Solid Edge part; units mm, degrees
sketch "Sketch1" plane through (0, 0, 0) normal (0, -1, 0) x (1, 0, 0)
  circle A0 centre (0, 0) radius 1.5
extrude "Protrusion1" add sketch "Sketch1" against normal blind 16
sketch "Sketch2" plane through (0, 16, 0) normal (0, 1, 0) x (1, 0, 0)
  circle A0 centre (0, 0) radius 3
extrude "ExtrudedProtrusion_2" add sketch "Sketch2" along normal blind 2.52
sketch "Sketch3" plane through (0, 18.52, 0) normal (0, 1, 0) x (-1, 0, 0)
  line L0 (-2.9311, 0.6393) -> (2.9311, 0.6393)
  arc A0 (2.9311, 0.6393) -> (2.9311, -0.6393) centre (0, 0) cw
  line L1 (2.9311, -0.6393) -> (-2.9311, -0.6393)
  arc A1 (-2.9311, -0.6393) -> (-2.9311, 0.6393) centre (0, 0) cw
extrude "ExtrudedCutout_1" cut sketch "Sketch3" against normal blind 0.8
cosmetic_thread "Thread1"
properties material "Nylon, general purpose"
Geometry check sheet. Reference: the model listing, model coordinates, mm. A direction names the side the tool comes from. Give positions to 0.01 mm unless a question says otherwise; leave off trailing zeros. Loops run counter-clockwise (first coordinate to the right, second up) from the corner with the lowest first, then second, coordinate; pieces in that order, holes last.
(1) Section check A-A on z = 0. Record the cut outline in (x, y), then the cut area to 3 significant figures.
From the geometry:
outline: (-3, 16) - (-1.5, 16) - (-1.5, 0) - (1.5, 0) - (1.5, 16) - (3, 16) - (3, 17.72) - (-3, 17.72) - close
area: 58.3 mm2
(2) Section check B-B on x = 2.4. Record the cut outline in (y, z).
From the geometry:
outline: (16, -1.8) - (18.52, -1.8) - (18.52, -0.64) - (17.72, -0.64) - (17.72, 0.64) - (18.52, 0.64) - (18.52, 1.8) - (16, 1.8) - close
(3) Thickness scan on L1, parallel to Y at x = 2.7, z = 0.2; L2, parallel to Y at x = -0.2, z = 1.75; L3, parallel to Z at x = 0.1, y = 8.5. Record the ranges inside material, lowest first.
From the geometry:
L1: y = 16 to 17.72
L2: y = 16 to 18.52
L3: z = -1.5 to 1.5
(4) Release check for a two-part mould opening along Z. For faces 4 (the cylindrical face through (-1.5, 7.89, 0.07)), 5 (the flat face through (0, 18, -0.639)), 6 (the flat face through (0, 18.52, 2)) record: released by +Z, released by -Z, zero draft, split by the parting line, or undercut.
From the geometry:
face 4: split by the parting line
face 5: undercut
face 6: zero draft
(5) Depth check by flat-ended pin: pin 1 Ø2 at (y, z) = (7, -2) entering from -X; pin 2 Ø1 at (x, y) = (-1.5, 4.5) entering from +Z. Enter the tip coordinate at first touch or a pass-through.
From the geometry:
pin 1: stops at x = -1.12
pin 2: stops at z = 1.12
(6) Set-up check for faces 1 (the flat face through (-1.3, 16, 1.3)), 2 (the flat face through (0, 17.72, 0)), 3 (the flat face through (0, 18.52, -2)): record each of +Z, -Z, +X, -X, +Y, -Y from which the full face is reachable in a straight line by a thin tool's end or side.
From the geometry:
face 1: -Y
face 2: +X, -X, +Y
face 3: +Z, -Z, +X, -X, +Y
(7) Section check C-C on y = 8.25. Record the cut outline in (x, z), then the cut area to 3 significant figures.
From the geometry:
outline: circle Ø3 at (0, 0)
area: 7.07 mm2
(8) Section check D-D on x = 0. Record the cut outline in (y, z), then the cut area to 3 significant figures.
From the geometry:
outline: (0, -1.5) - (16, -1.5) - (16, -3) - (18.52, -3) - (18.52, -0.64) - (17.72, -0.64) - (17.72, 0.64) - (18.52, 0.64) - (18.52, 3) - (16, 3) - (16, 1.5) - (0, 1.5) - close
area: 62.1 mm2
